Input: part model. Units: mm. Frame: model coordinates. A direction names the side the tool comes from. Coordinates: 2 decimals unless noted, no trailing zeros. Order: outer loops, then holes, each group sorted by start corner. A loop starts at its lowest first (then second) coordinate and runs counter-clockwise, first axis right, second up. Notation, with made-up numbers: (-23, 23) -> (25, 23) arc R4 ccw to (25, 28) -> close; hole circle Ø4 at (41, 82). An arc over 180 degrees is marked (long way). Use CSV: the item, a comma, the result in double quotes. Start each with the question number.
```python
from build123d import *

# Parameters (mm, degrees)
BOSS_EXTRUDE1_DEPTH = 4.95
SKETCH2_R           = 2.05
CUT_EXTRUDE1_DEPTH  = 179.606105426
BOSS_EXTRUDE2_START = 2
SKETCH4_R           = 2.05
BOSS_EXTRUDE2_DEPTH = 2
SKETCH5_R           = 3.375
CUT_EXTRUDE2_DEPTH  = 3
FILLET1_R           = 1


with BuildPart() as part:
    # Sketch1 → Boss-Extrude1 (new body)
    with BuildSketch(Plane(origin=(0, -273.846152423, 0), x_dir=(-1, 0, 0), z_dir=(0, -1, 0))):
        Polygon((82.019978644, 71.058996872), (82.302821357, 71.341839584), (89.377289978, 78.416308206), (91.393147439, 85.939590671), (85.940417335, 91.392320775), (78.41713487, 89.376463314), (71.342666248, 82.301994692), (71.059823536, 82.01915198), (26.834314575, 126.244660941), (-26.834314575, 126.244660941), (-71.058996872, 82.019978644), (-71.341839584, 82.302821357), (-78.416308206, 89.377289978), (-85.939590671, 91.393147439), (-91.392320775, 85.940417335), (-89.376463314, 78.41713487), (-82.301994692, 71.342666248), (-82.01915198, 71.059823536), (-126.244660941, 26.834314575), (-126.244660941, -26.834315555), (-82.020164054, -71.059182282), (-82.302821357, -71.341839584), (-89.377289978, -78.416308206), (-91.393147439, -85.939590671), (-85.940417335, -91.392320775), (-78.41713487, -89.376463314), (-71.342666248, -82.301994692), (-71.060054774, -82.019383219), (-26.834316916, -126.245490927), (26.834310282, -126.245490927), (71.059226271, -82.020208043), (71.341839584, -82.302821357), (78.416308206, -89.377289978), (85.939590671, -91.393147439), (91.392320775, -85.940417335), (89.376463314, -78.41713487), (82.301994692, -71.342666248), (82.019335916, -71.060007471), (126.244660941, -26.834315547), (126.244660941, 26.834314575), align=None)
        Polygon((-32.999177325, -28.496194078), (-32.999177325, -5.25), (-32.999177325, 5.25), (-32.999177325, 28.496194078), (-27.095371402, 34.4), (31.271815024, 34.4), (47.175620946, 18.496194078), (47.175620946, -18.496194078), (21.271815024, -44.4), (-17.095371403, -44.4), align=None, mode=Mode.SUBTRACT)
    extrude(amount=-BOSS_EXTRUDE1_DEPTH)

    # Sketch2 → Cut-Extrude1 (cut, through all)
    with BuildSketch(Plane(origin=(0, -268.896152423, 0), x_dir=(1, 0, 0), z_dir=(0, 1, 0))):
        with Locations(Location((-86.015131958, 86.014305294, 0), (0, 0, 180))):
            Circle(SKETCH2_R)
        with Locations(Location((86.014305294, 86.015131958, 0), (0, 0, 180))):
            Circle(SKETCH2_R)
        with Locations(Location((86.015135278, -86.01513528, 0), (0, 0, 180))):
            Circle(SKETCH2_R)
        with Locations(Location((-86.015036236, -86.015036236, 0), (0, 0, 180))):
            Circle(SKETCH2_R)
        with Locations(Location((1.349177325, 53.85640646, 0), (0, 0, 180))):
            Circle(SKETCH2_R)
        with Locations(Location((-52.507229136, 0, 0), (0, 0, 180))):
            Circle(SKETCH2_R)
        with Locations(Location((1.349177325, -53.856406461, 0), (0, 0, 180))):
            Circle(SKETCH2_R)
    extrude(amount=-CUT_EXTRUDE1_DEPTH, mode=Mode.SUBTRACT)

    # Sketch4 → Boss-Extrude2 (add)
    # profile 1 of 3: a face of its own
    with BuildSketch(Plane(origin=(0, -268.896152423, 0), x_dir=(1, 0, 0), z_dir=(0, 1, 0)).offset(BOSS_EXTRUDE2_START)):
        Polygon((17.099177325, 47.933012702), (17.099177325, 34.65), (-14.400822675, 34.65), (-14.400822675, 47.933012702), (-6.506485108, 61.60640646), (9.204839757, 61.60640646), align=None)
        with Locations(Location((1.349177325, 53.85640646, 0), (0, 0, 180))):
            Circle(SKETCH4_R, mode=Mode.SUBTRACT)
    # profile 2 of 3: a face of its own
    with BuildSketch(Plane(origin=(0, -268.896152423, 0), x_dir=(1, 0, 0), z_dir=(0, 1, 0)).offset(BOSS_EXTRUDE2_START)):
        Polygon((-60.257229136, 7.855662432), (-60.257229136, -7.855662433), (-47.425620946, -15.263994875), (-47.425620946, 15.263994875), align=None)
        with Locations(Location((-52.507229136, 0, 0), (0, 0, 180))):
            Circle(SKETCH4_R, mode=Mode.SUBTRACT)
    # profile 3 of 3: a face of its own
    with BuildSketch(Plane(origin=(0, -268.896152423, 0), x_dir=(1, 0, 0), z_dir=(0, 1, 0)).offset(BOSS_EXTRUDE2_START)):
        Polygon((-14.400822675, -44.65), (17.099177325, -44.65), (17.099177325, -47.933012702), (9.204839758, -61.606406461), (-6.506485108, -61.606406461), (-14.400822675, -47.933012702), align=None)
        with Locations(Location((1.349177325, -53.856406461, 0), (0, 0, 180))):
            Circle(SKETCH4_R, mode=Mode.SUBTRACT)
    extrude(amount=-BOSS_EXTRUDE2_DEPTH)

    # Sketch5 → Cut-Extrude2 (cut)
    with BuildSketch(Plane.XZ.offset(273.846152423)):
        with Locations(Location((1.349177325, 53.856406461, 0), (0, 0, 270))):
            Circle(SKETCH5_R)
        with Locations(Location((-52.507229136, 0, 0), (0, 0, 270))):
            Circle(SKETCH5_R)
        with Locations(Location((1.349177325, -53.85640646, 0), (0, 0, 270))):
            Circle(SKETCH5_R)
        with BuildLine():
            Line((83.628649892, 88.401620667), (86.279883668, 91.052854443))
            Line((86.279883668, 91.052854443), (91.052854441, 86.27988367))
            Line((91.052854441, 86.27988367), (88.401620665, 83.628649894))
            ThreePointArc((88.401620665, 83.628649894), (83.628649892, 83.628649894), (83.628649892, 88.401620667))
        make_face()
        with BuildLine():
            Line((88.401620667, -83.628649892), (91.052854443, -86.279883668))
            Line((91.052854443, -86.279883668), (86.27988367, -91.052854441))
            Line((86.27988367, -91.052854441), (83.628649894, -88.401620665))
            ThreePointArc((83.628649894, -88.401620665), (83.628649894, -83.628649892), (88.401620667, -83.628649892))
        make_face()
        with BuildLine():
            Line((-83.628649892, -88.401620667), (-86.279883668, -91.052854443))
            Line((-86.279883668, -91.052854443), (-91.052854441, -86.27988367))
            Line((-91.052854441, -86.27988367), (-88.401620665, -83.628649894))
            ThreePointArc((-88.401620665, -83.628649894), (-83.628649892, -83.628649894), (-83.628649892, -88.401620667))
        make_face()
        with BuildLine():
            Line((-88.401620667, 83.628649892), (-91.052854443, 86.279883668))
            Line((-91.052854443, 86.279883668), (-86.27988367, 91.052854441))
            Line((-86.27988367, 91.052854441), (-83.628649894, 88.401620665))
            ThreePointArc((-83.628649894, 88.401620665), (-83.628649894, 83.628649892), (-88.401620667, 83.628649892))
        make_face()
    extrude(amount=-CUT_EXTRUDE2_DEPTH, mode=Mode.SUBTRACT)

    # Fillet1
    # the kernel refuses this fillet: 1 mm, written as the material it takes off along each edge
    with BuildSketch(Plane(origin=(86.27988367, -275.983462791, -91.052854441), x_dir=(-0.7071067811867837, 0, -0.7071067811863112), z_dir=(0, 1, 0)), Plane(origin=(-91.052854441, -275.983462791, -86.27988367), x_dir=(-0.7071067811863703, 0, 0.7071067811867247), z_dir=(0, 1, 0)), Plane(origin=(-86.27988367, -275.983462791, 91.052854441), x_dir=(0.7071067811867394, 0, 0.7071067811863555), z_dir=(0, 1, 0)), Plane(origin=(91.052854441, -275.983462791, 86.27988367), x_dir=(0.7071067811863704, 0, -0.7071067811867248), z_dir=(0, 1, 0))) as fillet1_piece_1:
        with BuildLine():
            CenterArc((1, 0.854924147), FILLET1_R, 180, 58.751355935)
            Line((0, 0.854924147), (-0.02, 0.854924147))
            Line((-0.02, 0.854924147), (-0.02, 0))
            Line((-0.02, 0), (0, -0.02))
            ThreePointArc((0, -0.02), (0.240623487, -0.02), (0.470871913, -0.017098483))
            Line((0.470871913, -0.017098483), (0.481246974, 0))
        make_face()
    extrude(amount=5.137310369, mode=Mode.SUBTRACT)
    with BuildSketch(Plane(origin=(91.052854443, -275.981686608, -86.279883668), x_dir=(0.7071067811863996, 0, 0.7071067811866956), z_dir=(0, 1, 0)), Plane(origin=(-86.279883668, -275.981686608, -91.052854443), x_dir=(0.7071067811866807, 0, -0.7071067811864143), z_dir=(0, 1, 0)), Plane(origin=(-91.052854443, -275.981686608, 86.279883668), x_dir=(-0.7071067811863847, 0, -0.7071067811867103), z_dir=(0, 1, 0)), Plane(origin=(86.279883668, -275.981686608, 91.052854443), x_dir=(-0.7071067811866955, 0, 0.7071067811863995), z_dir=(0, 1, 0))) as fillet1_piece_2:
        with BuildLine():
            CenterArc((1, -0.854213674), FILLET1_R, 121.327026837, 58.672973163)
            Line((0, -0.854213674), (-0.02, -0.854213674))
            Line((-0.02, -0.854213674), (-0.02, 0))
            Line((-0.02, 0), (0, 0.02))
            ThreePointArc((0, 0.02), (0.240038946, 0.02), (0.469679449, 0.017084273))
            Line((0.469679449, 0.017084273), (0.480077891, 0))
        make_face()
    extrude(amount=5.135534185, mode=Mode.SUBTRACT)


solid = part.part
```
1. Section A-A on x = -17.5. Return loops of the section in (y, z).
2. Material intervals for line 1 along Z through (x, y) = (-17.5, -270.25); line 2 along Z through (x, y) = (2.5, -272.25); line 3 along Z through (x, y) = (5, -268.75), sorted ascending.
3. Section C-C on z = 66. Return loops of the section in (x, y), then the cut area to 3 significant figures.
4. Access query for faces 1 (the face through (-10.398, -267.882, 54.865)), 2 (the face through (-88.4, -270.846, 86.1)), 3 (the face through (48.64, -271.41, -104.44)), 4 (the face through (85.75, -271.41, -74.79)), 5 (the face through (30.089, -271.406, -31.407)). Directions: +Z, -Z, +X, -X, +Y, -Y. A direction counts if a zero-diameter tool reaches every point of the face in a straight line with its end or side. Return the directions, or none.
5. Contact query for flat-ended pins moving along their axis: P1, Ø5.5, axis at x = 2, z = -53.5, coming from the -Y side; P2, Ø4, axis at x = 1.35, z = 53.86, coming from the +Y side; P3, Ø0.6, axis at y = -268, z = -39.5, coming from the +X side; P4, Ø3, axis at y = -270.5, z = -93.5, coming from the -X side. Output: stop coordinate, or through.
6. Section B-B on z = -108.5. Return loops of the section in (x, y).
7. Pull-direction query (Z, two-part tool) for faces 6 (the face through (13.21, -267.88, 54.67)), 7 (the face through (83.58, -272.37, -83.68)), 8 (the face through (-74.79, -271.41, -85.75)); classes: released by +Z, released by -Z, zero draft, split by the parting line, or undercut.
Values follow:
1,outline,"(-273.85, -126.24) -> (-268.9, -126.24) -> (-268.9, -34.4) -> (-273.85, -34.4) -> close; (-273.85, 44.4) -> (-268.9, 44.4) -> (-268.9, 126.25) -> (-273.85, 126.25) -> close"
2,line 1,"z = -126.24 to -34.4, 44.4 to 126.25"
2,line 2,"z = -126.24 to -57.03, -50.68 to -34.4, 44.4 to 50.68, 57.03 to 126.25"
2,line 3,"z = -61.61 to -34.65, 44.65 to 61.61"
3,outline,"(-87.08, -273.85) -> (87.08, -273.85) -> (87.08, -268.9) -> (-87.08, -268.9) -> close"
3,area,"862 mm2"
4,face 1,"+Z, -X, +Y"
4,face 2,"-Y"
4,face 3,"-Z, +Y, -Y"
4,face 4,"+X, +Y, -Y"
4,face 5,"+Y, -Y"
5,P1,"stops at y = -273.85"
5,P2,"passes through"
5,P3,"stops at x = 17.1"
5,P4,"stops at x = -61.08"
6,outline,"(-44.58, -273.85) -> (44.58, -273.85) -> (44.58, -268.9) -> (-44.58, -268.9) -> close"
7,face 6,"released by +Z"
7,face 7,"undercut"
7,face 8,"released by -Z"
